```python
from build123d import *

# Parameters (mm, degrees)
SKETCH1_R           = 17.907
BOSS_EXTRUDE1_DEPTH = 53.34
SKETCH2_OUTSIDE_W   = 55.452
SKETCH2_OUTSIDE_H   = 55.452
SKETCH2_OUTSIDE_R   = 9.906
CUT_EXTRUDE1_DEPTH  = 41.91
CUT_EXTRUDE1_DRAFT  = -2
FILLET1_R           = 1.27
FILLET2_R           = 3.81
FILLET3_R           = 2.54
SKETCH4_R           = 2.54
BOSS_EXTRUDE3_DEPTH = 28.067
FILLET4_R           = 1.27


with BuildPart() as part:
    # Sketch1 → Boss-Extrude1 (new body)
    with BuildSketch(Plane(origin=(0, 0, 0), x_dir=(1, 0, 0), z_dir=(0, 1, 0))):
        with Locations(Location((0, 0, 0), (0, 0, 270))):
            Circle(SKETCH1_R)
    extrude(amount=BOSS_EXTRUDE1_DEPTH)


with BuildPart() as cut_extrude1_tool:
    # Sketch2 outside → Cut-Extrude1 (with draft: the straight prism first)
    with BuildSketch(Plane(origin=(0, 11.43, 0), x_dir=(1, 0, 0), z_dir=(0, 1, 0))):
        Rectangle(SKETCH2_OUTSIDE_W, SKETCH2_OUTSIDE_H)
        Circle(SKETCH2_OUTSIDE_R, mode=Mode.SUBTRACT)
    extrude(amount=CUT_EXTRUDE1_DEPTH)
    # Cut-Extrude1: the draft: its side faces are tilted about the plane it starts from
    cut_extrude1_sides = [cut_extrude1_tool.faces().sort_by_distance(p)[0] for p in [
        (0, 32.385, 27.726),
        (27.726, 32.385, 0),
        (0, 32.385, -27.726),
        (-27.726, 32.385, 0),
        (-9.906, 32.385, 0),
    ]]
    draft(cut_extrude1_sides, Plane(origin=(0, 11.43, 0), x_dir=(1, 0, 0), z_dir=(0, 1, 0)), CUT_EXTRUDE1_DRAFT)


with BuildPart() as part_1:
    add(part.part)

    # Cut-Extrude1: cut by cut_extrude1_tool
    add(cut_extrude1_tool.part, mode=Mode.SUBTRACT)

    # Fillet1
    fillet1_edges = [part_1.edges().sort_by_distance(p)[0] for p in [
        (-8.442470551, 53.34, 0),
    ]]
    fillet(fillet1_edges, radius=FILLET1_R)

    # Fillet2
    fillet2_edges = [part_1.edges().sort_by_distance(p)[0] for p in [
        (0, 11.43, -17.907),
    ]]
    fillet(fillet2_edges, radius=FILLET2_R)

    # Fillet3
    fillet3_edges = [part_1.edges().sort_by_distance(p)[0] for p in [
        (-9.906, 11.43, 0),
    ]]
    fillet(fillet3_edges, radius=FILLET3_R)

    # Sketch4 → Boss-Extrude3 (add)
    with BuildSketch(Plane.XY):
        with Locations((0, 3.81)):
            Circle(SKETCH4_R)
    extrude(amount=-BOSS_EXTRUDE3_DEPTH)

    # Fillet4
    fillet4_edges = [part_1.edges().sort_by_distance(p)[0] for p in [
        (-2.54, 3.81, -28.067),
    ]]
    fillet(fillet4_edges, radius=FILLET4_R)


solid = part_1.part
```
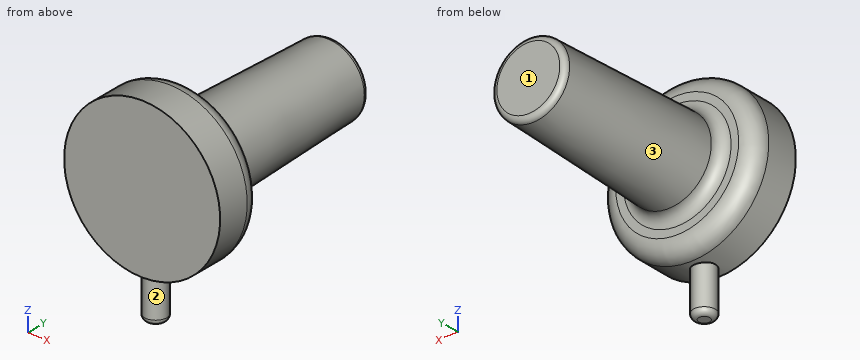
Design review of the part built by this model. Coordinates are the model's own, in mm. Face numbers are marked on the shaded views. A direction names the side the tool comes from. Coordinates: 2 decimals unless noted, no trailing zeros. Order: outer loops, then holes, each group sorted by start corner. A loop starts at its lowest first (then second) coordinate and runs counter-clockwise, first axis right, second up. Notation, with made-up numbers: (-18, 75.5) - (-6, 75.5) arc R16 ccw to (-6, 85.5) - close; hole circle Ø5 at (1.5, 21). An arc over 180 degrees is marked (long way). One line per question, with ' | ' between items.
Q1. Consider section C-C, the plane z = -21. Give the boundary of the cut face in (x, y), then the cut area to 3 significant figures.
Answer key:
outline: circle Ø5.08 at (0, 3.81) | area: 20.3 mm2
Q2. Consider section A-A, the plane z = 0. Give the boundary of the cut face in (x, y).
Answer key:
outline: (-17.91, 0) - (17.91, 0) - (17.91, 7.62) arc R3.81 ccw to (14.1, 11.43) - (12.36, 11.43) arc R2.54 cw to (9.82, 13.88) - (8.49, 52.11) arc R1.27 ccw to (7.22, 53.34) - (-7.22, 53.34) arc R1.27 ccw to (-8.49, 52.11) - (-9.82, 13.88) arc R2.54 cw to (-12.36, 11.43) - (-14.1, 11.43) arc R3.81 ccw to (-17.91, 7.62) - close
Q3. For the marked faces 1, 2 and 3, list the 3-axis set-ups (+Z, -Z, +X, -X, +Y, -Y) from which the entire face can be reached by the end or side of a thin tool; tool diameter is ignored.
Answer key:
face 1: +Z, -Z, +X, -X, +Y | face 2: -Z | face 3: +Y
Q4. To check wall thickness, follow line 1 along Y through (x, z) = (8, -12); line 2 along Z through (x, y) = (-7, 43.5); line 3 along Y through (x, z) = (4.5, -7). State the ranges of each line that lie inside material, in increasing order.
Answer key:
line 1: y = 0 to 11.42 | line 2: z = -5.31 to 5.31 | line 3: y = 0 to 52.69
Q5. Consider section B-B, the plane y = 18. Give the boundary of the cut face in (x, z), then the cut area to 3 significant figures.
Answer key:
outline: circle Ø19.35 at (0, 0) | area: 294 mm2
Q6. Clearance check with flat-ended pins moving along their axes: pin 1 Ø12 at (x, y) = (-14, 25) entering from -Z; pin 2 Ø8 at (x, y) = (14.5, 9) entering from -Z; pin 3 Ø4 at (x, y) = (13, 25) entering from -Z; pin 4 Ø1.5 at (x, z) = (-5.5, -11.5) entering from +Y. State where each tip first meets the part, or that it passes through.
Answer key:
pin 1: stops at z = -5 | pin 2: stops at z = -14.39 | pin 3: passes through | pin 4: stops at y = 11.46
